Design review of the part built by this model. Coordinates are the model's own, in mm. A direction names the side the tool comes from. Round coordinates to 2 decimals unless told otherwise and drop trailing zeros. Loops run counter-clockwise (first coordinate to the right, second up) from the corner with the lowest first, then second, coordinate; pieces in that order, holes last. Notation, with made-up numbers: M 8.5,11.25 L 64.5,11.25 A13 cw 64.5,16.25 Z; hole C 69.25,26 d10. An arc over 180 degrees is marked long. One line per item, written item: value. Start each with the question number.
Item 1: We need section A-A (x = 0). Write out the cut boundary in (y, z), then the cut area to 3 significant figures.
Item 2: Mouldability with a two-part tool opening along Y and no side actions: class faces 1 (the cylindrical face through (1.099, 0.012, -0.21)), 2 (the flat face through (1, 104.16, 0)), 3 (the flat face through (-80, 99, 0)), 4 (the cylindrical face through (-5.42, 25.594, 0.21)) as released by +Y, released by -Y, zero draft, split by the parting line, or undercut.
Item 3: We need section D-D (x = -57). Write out the cut boundary in (y, z), then the cut area to 3 significant figures.
Item 4: Clearance check with flat-ended pins moving along their axes: pin 1 (10 mm diameter, centred on y = 74, z = -3, fed in from +X); pin 2 (9 mm diameter, centred on x = -68, z = -6, fed in from -Y); pin 3 (2 mm diameter, centred on y = 15.5, z = -5, fed in from -X); pin 4 (2 mm diameter, centred on x = 51, y = 44, fed in from +Z). State where each tip first meets the part, or that it passes through.
Item 5: We need section C-C (y = 92). Write out the cut boundary in (x, z).
Item 6: For line 1 along Y through (x, z) = (0, 4.25); line 2 along X through (y, z) = (49.5, -12.5) (1 decimal); line 3 along X through (y, z) = (79, 3), list the stretches that pass through material, from the lowest coordinate up.
Item 7: For faces 5 (the flat face through (80, 99, 0)), 6 (the flat face through (-65, 94.67, 0)), 7 (the flat face through (65, 94.67, 0)), list the 3-axis set-ups (+Z, -Z, +X, -X, +Y, -Y) from which the entire face can be reached by the end or side of a thin tool; tool diameter is ignored.
Item 8: We need section B-B (z = 3.5). Write out the cut boundary in (x, y), then the cut area to 3 significant figures.
Autodesk Inventor part; units mm, degrees
ref_plane "YZ Plane" through (0, 0, 0) normal (1, 0, 0) x (0, 1, 0)
ref_plane "XZ Plane" through (0, 0, 0) normal (0, 1, 0) x (-1, 0, 0)
ref_plane "XY Plane" through (0, 0, 0) normal (0, 0, 1) x (1, 0, 0)
sketch "Sketch1" plane through (0, 0, 0) normal (0, 0, 1) x (1, 0, 0)
  arc A0 (-50, 50) -> (0, 0) centre (0, 50) ccw
  line L0 (0, 0) -> (0, 52.848) construction
  line L1 (0, 0) -> (-10.7104, 0) construction
  arc A1 (0, 0) -> (50, 50) centre (0, 50) ccw
  circle A2 centre (0, 50) radius 25
  arc A3 (0, 25) -> (25, 50) centre (0, 50) ccw
  line L2 (-50, 50) -> (-50, 85)
  line L3 (50, 50) -> (50, 85)
  line L4 (50, 85) -> (-50, 85)
  dimension "d0" = 50
  dimension "d1" = 25
  dimension "d15" = 85
extrude "Extrusion1" add sketch "Sketch1" along normal mid plane 30
sketch "Sketch5" plane through (-50, 85, 15) normal (0, 1, 0) x (1, 0, 0)
  line L0 (100, 30) -> (100, 0)
  line L1 (100, 30) -> (130, 30)
  line L2 (130, 30) -> (130, 0)
  line L3 (130, 0) -> (100, 0)
  line L4 (100, 0) -> (100, 30)
  line L5 (0, 30) -> (0, 0)
  line L6 (0, 30) -> (-30, 30)
  line L7 (-30, 30) -> (-30, 0)
  line L8 (-30, 0) -> (0, 0)
  line L9 (0, 0) -> (0, 30)
  point P0 (50, 15)
  dimension "d16" = 30
  dimension "d17" = 30
  dimension "d18" = 30
  dimension "d19" = 30
extrude "Extrusion4" add sketch "Sketch5" against normal blind 6
move faces "Move1" translate (0, 25.99, 0) faces at (-26.6667, 85, -5)
move faces "Move2" translate (0, 22.5, 0) faces at (-70, 79, -5) (60, 79, -5)
move faces "Move3" translate (0, -6.83, 0) faces at (1.0045, 92.6059, 15) (1.0045, 92.6059, -15) (26.6667, 110.99, 5) (-80, 107.8267, -5) (80, 107.8267, 5) (60, 101.5, -5) (-70, 101.5, -5)
properties part number "wheel holder"
A:
1. outline: M 0,-15 L 25,-15 L 25,15 L 0,15 Z; M 75,-15 L 104.16,-15 L 104.16,15 L 75,15 Z
1. area: 1,620 mm2
2. face 1: released by -Y
2. face 2: released by +Y
2. face 3: zero draft
2. face 4: undercut
3. outline: M 94.67,-15 L 104.16,-15 L 104.16,15 L 94.67,15 Z
3. area: 285 mm2
4. pin 1: x = 50
4. pin 2: y = 94.67
4. pin 3: x = -37.12
4. pin 4: through
5. outline: M -50,-15 L 50,-15 L 50,15 L -50,15 Z
6. line 1: 0 to 25, 75 to 104.16
6. line 2: -50 to -25, 25 to 50
6. line 3: -50 to 50
7. face 5: +Z, -Z, +X, +Y, -Y
7. face 6: +Z, -Z, -X, -Y
7. face 7: +Z, -Z, +X, -Y
8. outline: M -80,94.67 L -50,94.67 L -50,50 A50 ccw 50,50 L 50,94.67 L 80,94.67 L 80,104.16 L -80,104.16 Z; hole C 0,50 d50
8. area: 7,950 mm2
